CAD build for the part. Positions are in the model's coordinates, mm. A direction names the side the tool comes from. Give positions to 0.01 mm unless a question says otherwise; leave off trailing zeros. Loops run counter-clockwise (first coordinate to the right, second up) from the corner with the lowest first, then second, coordinate; pieces in that order, holes last.
Item 1: Saw through at A-A on z = 29. Give the cut face in (x, y).
Item 2: Probe probe 1 along X at (y, z) = (-18, 6); probe 2 along Y at (x, z) = (16, 12); probe 3 along X at (y, z) = (-6.5, 7). List the from-to ranges inside material, lowest first.
Item 3: Saw through at C-C on x = -2.5. Give the cut face in (y, z).
Item 4: Which spindle directions (+Z, -Z, +X, -X, +Y, -Y) get a long thin tool onto all of the face, cutting with end or side? Do faces 4 (the flat face through (0, -35, 10)), 5 (the flat face through (30, -44, 25)), 6 (the flat face through (35, 37, 25)), 7 (the flat face through (18, 1, 10)). Say none if no direction does.
Item 5: Saw through at D-D on x = 9. Give the cut face in (y, z).
Item 6: Saw through at B-B on y = 1. Give the cut face in (x, z), plus the area to 3 significant figures.
Item 7: Mould opens along Y. For faces 1 (the flat face through (-40, -1, 12)), 2 (the flat face through (36, 0, 17)), 3 (the flat face through (-0.6, -50, 9.5)) say: released by +Y, released by -Y, zero draft, split by the parting line, or undercut.
Item 8: Drop flat-ended pins along their axis: P1, Ø10.5, axis at x = -5.5, z = 34.5, coming from the -Y side; P2, Ø10, axis at x = 12, y = 9, coming from the +Z side; P3, Ø6.5, axis at x = -35, y = 5.5, coming from the +Z side. Give the stop position or say it passes through.
from build123d import *

# Parameters (mm, degrees)
SKETCH_W        = 80
SKETCH_H        = 100
PAD_DEPTH       = 25
SKETCH001_W     = 64
SKETCH001_H     = 84
POCKET_DEPTH    = 15
SKETCH002_W     = 10
SKETCH002_H     = 27.891991
POCKET001_DEPTH = 100.001
SKETCH003_W     = 30
SKETCH003_H     = 18.544697
POCKET002_DEPTH = 80.001
PAD001_DEPTH    = 8
POCKET003_DEPTH = 10


with BuildPart() as part:
    # Sketch → Pad (new body)
    with BuildSketch(Plane.XY):
        Rectangle(SKETCH_W, SKETCH_H)
    extrude(amount=PAD_DEPTH)

    # Sketch001 → Pocket (cut)
    with BuildSketch(Plane.XY.offset(25)):
        Rectangle(SKETCH001_W, SKETCH001_H)
    extrude(amount=-POCKET_DEPTH, mode=Mode.SUBTRACT)

    # Sketch002 → Pocket001 (cut, through all)
    with BuildSketch(Plane.XZ.offset(50)):
        with Locations((0, 23.945995)):
            Rectangle(SKETCH002_W, SKETCH002_H)
    extrude(amount=-POCKET001_DEPTH, mode=Mode.SUBTRACT)

    # Sketch003 → Pocket002 (cut, through all)
    with BuildSketch(Plane.YZ.offset(40)):
        with Locations((0, 26.272348)):
            Rectangle(SKETCH003_W, SKETCH003_H)
    extrude(amount=-POCKET002_DEPTH, mode=Mode.SUBTRACT)

    # Sketch004 → Pad001 (new body)
    with BuildSketch(Plane(origin=(0, 50, 0), x_dir=(-1, 0, 0), z_dir=(0, 1, 0))):
        Polygon((12, 25), (12, 45), (-12, 45), (-12, 25), (-5, 25), (-5, 37), (5, 37), (5, 25), align=None)
    extrude(amount=-PAD001_DEPTH)

    # Sketch005 → Pocket003 (cut)
    with BuildSketch(Plane.XY.offset(10)):
        Polygon((-7.5, 10), (-7.5, 20), (7.5, 20), (7.5, 10), (12.5, 10), (12.5, -10), (7.5, -10), (7.5, -20), (-7.5, -20), (-7.5, -10), (-12.5, -10), (-12.5, 10), align=None)
    extrude(amount=-POCKET003_DEPTH, mode=Mode.SUBTRACT)


solid = part.part
Results below:
1. outline: (-12, 42) - (-5, 42) - (-5, 50) - (-12, 50) - close; (5, 42) - (12, 42) - (12, 50) - (5, 50) - close
2. probe 1: x = -40 to -7.5, 7.5 to 40
2. probe 2: y = -50 to -42, 42 to 50
2. probe 3: x = -40 to -12.5, 12.5 to 40
3. outline: (-50, 0) - (-20, 0) - (-20, 10) - (-50, 10) - close; (20, 0) - (50, 0) - (50, 10) - (20, 10) - close; (42, 37) - (50, 37) - (50, 45) - (42, 45) - close
4. face 4: +Z, +Y, -Y
4. face 5: +Z, +X, -X, -Y
4. face 6: +Z, +X, +Y, -Y
4. face 7: +Z
5. outline: (-50, 0) - (-10, 0) - (-10, 10) - (-42, 10) - (-42, 25) - (-50, 25) - close; (10, 0) - (50, 0) - (50, 45) - (42, 45) - (42, 10) - (10, 10) - close
6. outline: (-40, 0) - (-12.5, 0) - (-12.5, 10) - (-32, 10) - (-32, 17) - (-40, 17) - close; (12.5, 0) - (40, 0) - (40, 17) - (32, 17) - (32, 10) - (12.5, 10) - close
6. area: 662 mm2
7. face 1: zero draft
7. face 2: undercut
7. face 3: released by -Y
8. P1: stops at y = 42
8. P2: stops at z = 10
8. P3: stops at z = 17
